For this review, take the finished solid that the model builds, in its own axes (mm). A direction names the side the tool comes from. Round coordinates to 2 decimals unless told otherwise and drop trailing zeros. Order: outer loops, then holes, each group sorted by start corner. A loop starts at its lowest first (then second) coordinate and runs counter-clockwise, first axis right, second up. Notation, with made-up numbers: (1.25, 24.5) - (21.25, 24.5) arc R22 cw to (21.25, 52.5) - close; hole circle Ø4 at (83, 77). An arc over 180 degrees is marked (long way). Write each question's results on one line, items separated by ' | '. Start each with the question number.
(1) For L1, parallel to Z at x = 0, y = 14.3; L2, parallel to X at y = 16.55, z = 0; L3, parallel to Z at x = 0, y = 16.75, list the stretches that pass through material, from the lowest coordinate up. Write a range as from..to.
(2) Draft analysis for pull direction X (two halves, no side actions). For faces 3 (the cylindrical face through (-10.3, 15.5, 0.6)), 4 (the flat face through (0, 0, 0)), 5 (the cylindrical face through (-1.5, 20.96, 0.07)), 6 (the flat face through (9, 13, 0)), state which applies: pulls with the +X half, pulls with the -X half, needs draft (parallel to the pull), parting line crosses it, or undercut.
(3) Take a section at A-A, the plane y = 15.5. Give the boundary of the cut face in (x, z), plus the area to 3 significant figures.
(4) Take a section at B-B, the plane z = 0. Give the boundary of the cut face in (x, y).
(5) For faces 1 (the flat face through (-10, 13, 0)), 2 (the cylindrical face through (-12.932, 6.409, 5.362)), list the 3-axis set-ups (+Z, -Z, +X, -X, +Y, -Y) from which the entire face can be reached by the end or side of a thin tool; tool diameter is ignored.
(6) Insertion check: pin 1 Ø8 at (y, z) = (3.5, -5) entering from -X; pin 2 Ø8 at (x, y) = (7.5, 10.5) entering from +Z; pin 3 Ø1.6 at (x, z) = (0.5, -8) entering from +Y. Each pin has a flat end and moves straight along its axis. Give the tip position at first contact, or say it passes through.
(7) Take a section at C-C, the plane y = 8. Give the boundary of the cut face in (x, z).
Autodesk Inventor part; units mm, degrees
ref_plane "YZ Plane" through (0, 0, 0) normal (1, 0, 0) x (0, 1, 0)
ref_plane "XZ Plane" through (0, 0, 0) normal (0, 1, 0) x (-1, 0, 0)
ref_plane "XY Plane" through (0, 0, 0) normal (0, 0, 1) x (1, 0, 0)
sketch "Эскиз1" plane through (0, 0, 0) normal (0, 1, 0) x (-1, 0, 0)
  circle A0 centre (0, 0) radius 14
  dimension "d0" = 28
extrude "Выдавливание1" add sketch "Эскиз1" along normal blind 18
sketch "Эскиз2" plane through (0, 18, 0) normal (0, 1, 0) x (1, 0, 0)
  circle A0 centre (0, 0) radius 1.5
  dimension "d3" = 3
extrude "Выдавливание2" add sketch "Эскиз2" along normal blind 6
sketch "Эскиз3" plane through (0, 18, 0) normal (0, 1, 0) x (1, 0, 0)
  circle A0 centre (0, 8) radius 1
  circle A1 centre (0, -8) radius 1
  circle A2 centre (-9.5, 0) radius 1
  circle A3 centre (9.5, 0) radius 1
  point P0 (0, 0)
  dimension "d6" = 2
  dimension "d7" = 2
  dimension "d8" = 2
  dimension "d9" = 2
  dimension "d10" = 8
  dimension "d11" = 8
  dimension "d12" = 9.5
  dimension "d13" = 9.5
extrude "Выдавливание3" cut sketch "Эскиз3" against normal blind 5
fillet "Сопряжение1" radius 5 1 edges at (14, 18, 0)
properties part number "motor_c2822"
Results below:
1) L1: z = -13.83..-9, -7..7, 9..13.83 | L2: x = -12.52..-10.5, -8.5..8.5, 10.5..12.52 | L3: z = -12.31..-9, -7..7, 9..12.31
2) face 3: undercut | face 4: needs draft | face 5: parting line crosses it | face 6: undercut
3) outline: circle Ø26.66 at (0, 0); hole circle Ø2 at (-9.5, 0); hole circle Ø2 at (0, -8); hole circle Ø2 at (0, 8); hole circle Ø2 at (9.5, 0) | area: 546 mm^2
4) outline: (-14, 0) - (14, 0) - (14, 13) arc R5 ccw to (10.5, 17.77) - (10.5, 13) - (8.5, 13) - (8.5, 18) - (1.5, 18) - (1.5, 24) - (-1.5, 24) - (-1.5, 18) - (-8.5, 18) - (-8.5, 13) - (-10.5, 13) - (-10.5, 17.77) arc R5 ccw to (-14, 13) - close
5) face 1: +Y | face 2: +Y, -Y
6) pin 1: stops at x = -13.96 | pin 2: stops at z = 13.56 | pin 3: stops at y = 18
7) outline: circle Ø28 at (0, 0)
